```python
from build123d import *

# Parameters (mm, degrees)
F0_R     = 6.35
F0_R_2   = 15.875
F1_DEPTH = 6.35


with BuildPart() as f1:
    # F0 (on Front) → F1 (new body)
    with BuildSketch(Plane.XZ):
        Polygon((-52.790296, 10.877535), (-52.790296, -33.572465), (48.809704, -33.572465), (48.809704, 10.877535), (9.553431, 33.566941), (-22.196569, 33.566941), align=None)
        with Locations((-33.740296, -14.522465)):
            Circle(F0_R, mode=Mode.SUBTRACT)
        with Locations((0, -1.822465)):
            Circle(F0_R_2, mode=Mode.SUBTRACT)
        with Locations((29.759704, -14.522465)):
            Circle(F0_R, mode=Mode.SUBTRACT)
    extrude(amount=F1_DEPTH)


solid = f1.part
```
For this review, take the finished solid that the model builds, in its own axes (mm). Round coordinates to 2 decimals unless told otherwise and drop trailing zeros. Order: outer loops, then holes, each group sorted by start corner. A loop starts at its lowest first (then second) coordinate and runs counter-clockwise, first axis right, second up.
Q1. Wall thickness on line 1 (X direction, y = -2.5, z = -1.5); line 2 (Z direction, x = 0, y = -1.25); line 3 (X direction, y = -2.75, z = -18.5): over which ranges is each line inside the solid? List them lowest first.
Findings below:
line 1: x = -52.79 to -15.87, 15.87 to 48.81
line 2: z = -33.57 to -17.7, 14.05 to 33.57
line 3: x = -52.79 to -38.69, -28.79 to 24.81, 34.71 to 48.81
Q2. Mouldability with a two-part tool opening along X and no side actions: class faces 1 (the flat face through (-6, -3, 33.567)), 2 (the cylindrical face through (24.721, -3.131, -18.386)), 3 (the flat face through (-37.28, -3.13, 22.38)) as pulls with the +X half, pulls with the -X half, needs draft (parallel to the pull), parting line crosses it, or undercut.
Findings below:
face 1: needs draft
face 2: undercut
face 3: pulls with the -X half
Q3. We need section C-C, the plane z = -16.5. Give the boundary of the cut face in (x, y).
Findings below:
outline: (-52.79, -6.35) - (-39.77, -6.35) - (-39.77, 0) - (-52.79, 0) - close; (-27.71, -6.35) - (-6.05, -6.35) - (-6.05, 0) - (-27.71, 0) - close; (6.05, -6.35) - (23.73, -6.35) - (23.73, 0) - (6.05, 0) - close; (35.79, -6.35) - (48.81, -6.35) - (48.81, 0) - (35.79, 0) - close
Q4. Insertion check: P1, Ø11.5, axis at x = -33.74, z = -14.52, coming from the +Y side. The pin has a flat end and moves straight along its axis. Give the tip position at first contact, or say it passes through.
Findings below:
P1: passes through
Q5. We need section D-D, the plane x = -33.5. Give the boundary of the cut face in (y, z).
Findings below:
outline: (-6.35, -33.57) - (0, -33.57) - (0, -20.87) - (-6.35, -20.87) - close; (-6.35, -8.18) - (0, -8.18) - (0, 25.18) - (-6.35, 25.18) - close
Q6. We need section B-B, the plane y = -5. Give the boundary of the cut face in (x, z) (3 decimals), plus the area to 3 significant figures.
Findings below:
outline: (-52.79, -33.572) - (48.81, -33.572) - (48.81, 10.878) - (9.553, 33.567) - (-22.197, 33.567) - (-52.79, 10.878) - close; hole circle Ø12.7 at (-33.74, -14.522); hole circle Ø31.75 at (0, -1.822); hole circle Ø12.7 at (29.76, -14.522)
area: 4,980 mm2
Q7. We need section A-A, the plane x = 0. Give the boundary of the cut face in (y, z).
Findings below:
outline: (-6.35, -33.57) - (0, -33.57) - (0, -17.7) - (-6.35, -17.7) - close; (-6.35, 14.05) - (0, 14.05) - (0, 33.57) - (-6.35, 33.57) - close
